Part model, mm, in its own coordinate system. A direction names the side the tool comes from. Round coordinates to 2 decimals unless told otherwise and drop trailing zeros. Loops run counter-clockwise (first coordinate to the right, second up) from the corner with the lowest first, then second, coordinate; pieces in that order, holes last. Notation, with made-up numbers: (-40, 44) -> (-28, 44) arc R27 ccw to (-28, 76) -> close; hole circle Ø3 at (-18, 36). An arc over 180 degrees is marked (long way). Use a Markdown table: item, result. Add a question column.
Item 1: Cut at D-D, the plane x = 10.5. List the corners of the cut face in (y, z).
Item 2: Which spindle directions (+Z, -Z, +X, -X, +Y, -Y) get a long thin tool onto all of the face, cutting with end or side? Do faces 4 (the face through (-10, -23, 46)), 5 (the face through (0, -33, 25)), 6 (the face through (7.5, -33, 13)). Say none if no direction does.
Item 3: Cut at A-A, the plane z = 35. List the corners of the cut face in (x, y).
Item 4: Cut at C-C, the plane y = -14. List the corners of the cut face in (x, z).
Item 5: Flat gauge pins, fed straight in: pin 1 (2 mm diameter, centred on x = 4, y = 8, fed in from +Z); pin 2 (22 mm diameter, centred on y = -36.5, z = 6.5, fed in from +X); pin 3 (4.5 mm diameter, centred on x = 10, z = 33, fed in from -Y). Where does each tip first touch, or does it go through?
Item 6: Probe line 1 (X direction, y = -18, z = 72.5); line 2 (Y direction, x = -7.5, z = 36); line 3 (Y direction, x = 11, z = 58). List the from-to ranges inside material, lowest first. Write a range as [from, to].
Item 7: Cut at B-B, the plane z = 62. List the corners of the cut face in (x, y).
Item 8: Two-plate mould, pull along X, no slides. Class faces 1 (the face through (-7.5, -33, 13)), 2 (the face through (0, -3, 0)), 3 (the face through (0, 21.5, 32)): pulls with the +X half, pulls with the -X half, needs draft (parallel to the pull), parting line crosses it, or undercut.
```python
from build123d import *

# Parameters (mm, degrees)
SKETCH_2_W          = 26
SKETCH_2_H          = 46
EXTRUDE_1_DEPTH     = 93
CUT_EXTRUDE_1_DEPTH = 8
SKETCH_7_W          = 25
SKETCH_7_H          = 20
EXTRUDE_2_DEPTH     = 7.5


with BuildPart() as part:
    # 스케치2 → 보스-돌출1 (new body)
    with BuildSketch(Plane.XY):
        Rectangle(SKETCH_2_W, SKETCH_2_H)
    extrude(amount=EXTRUDE_1_DEPTH)

    # 스케치3 → 컷-돌출1 (cut, symmetric)
    with BuildSketch(Plane(origin=(0, 0, 0), x_dir=(0, 0, -1), z_dir=(1, 0, 0))):
        Polygon((-93, -23), (-20, -23), (-20, 21.5), (-44.8, 21.5), (-44.8, 23), (-93, 23), align=None)
    extrude(amount=CUT_EXTRUDE_1_DEPTH, both=True, mode=Mode.SUBTRACT)

    # 스케치7 → 보스-돌출2 (add, symmetric)
    with BuildSketch(Plane(origin=(0, 0, 0), x_dir=(0, 0, -1), z_dir=(1, 0, 0))):
        with Locations((-12.5, -33)):
            Rectangle(SKETCH_7_W, SKETCH_7_H)
    extrude(amount=EXTRUDE_2_DEPTH, both=True)


solid = part.part
```
A:
| question | item | result |
|---|---|---|
| 1 | outline | (-23, 0) -> (23, 0) -> (23, 93) -> (-23, 93) -> close |
| 2 | face 4 | +Z, -Z, -X, -Y |
| 2 | face 5 | +Z, +X, -X, -Y |
| 2 | face 6 | +Z, -Z, +X, -Y |
| 3 | outline | (-13, -23) -> (-8, -23) -> (-8, 21.5) -> (8, 21.5) -> (8, -23) -> (13, -23) -> (13, 23) -> (-13, 23) -> close |
| 4 | outline | (-13, 0) -> (13, 0) -> (13, 93) -> (8, 93) -> (8, 20) -> (-8, 20) -> (-8, 93) -> (-13, 93) -> close |
| 5 | pin 1 | stops at z = 20 |
| 5 | pin 2 | stops at x = 7.5 |
| 5 | pin 3 | stops at y = -23 |
| 6 | line 1 | x = [-13, -8], [8, 13] |
| 6 | line 2 | y = [21.5, 23] |
| 6 | line 3 | y = [-23, 23] |
| 7 | outline | (-13, -23) -> (-8, -23) -> (-8, 23) -> (-13, 23) -> close; (8, -23) -> (13, -23) -> (13, 23) -> (8, 23) -> close |
| 8 | face 1 | pulls with the -X half |
| 8 | face 2 | needs draft |
| 8 | face 3 | undercut |
